```python
from build123d import *

# Parameters (mm, degrees)
F0_W     = 170
F0_H     = 170
F1_DEPTH = 40
F2_W     = 155
F2_H     = 113
F3_DEPTH = 17
F4_DEPTH = 24
F6_D     = 3.7973
F7_W     = 16.0088125554
F7_H     = 25.888455566
F7_W_2   = 40.4067277214
F7_H_2   = 12.8438859247
F7_W_3   = 24.2321552965
F7_H_3   = 26.0891397484
F7_W_4   = 19.8441686174
F7_H_4   = 32.3103985284
F8_DEPTH = 2


with BuildPart() as f1:
    # F0 (on Top) → F1 (new body)
    with BuildSketch(Plane.XY):
        Rectangle(F0_W, F0_H)
    extrude(amount=F1_DEPTH)

    # F2 (on face) → F3 (join)
    with BuildSketch(Plane.XY.offset(40)):
        with Locations((7.5, 1.5)):
            Rectangle(F2_W, F2_H)
    extrude(amount=F3_DEPTH)

    # F2 (on face) → F4 (cut)
    with BuildSketch(Plane.XY.offset(40)):
        Polygon((-70, 58), (-70, 85), (-85, 85), (-85, -85), (-70, -85), (-70, -55), align=None)
    extrude(amount=-F4_DEPTH, mode=Mode.SUBTRACT)

    # F6 (through all)
    with Locations(Plane(origin=(0, 0, 0), x_dir=(1, 0, 0), z_dir=(0, 0, -1))):
        with Locations((-78.65, -74.84), (78.83, -51.98), (78.83, 81.04), (-78.65, 81.04)):
            Hole(F6_D / 2)

    # F7 (on face) → F8 (join)
    with BuildSketch(Plane(origin=(0, 85, 0), x_dir=(-1, 0, 0), z_dir=(0, 1, 0))):
        with Locations((-71.7186613039, 17.3905782867)):
            Rectangle(F7_W, F7_H)
        with Locations((-35.5920631724, 10.868293466)):
            Rectangle(F7_W_2, F7_H_2)
        with Locations((7.3542475339, 17.4909203779)):
            Rectangle(F7_W_3, F7_H_3)
        with Locations((55.5439972199, 20.6015497679)):
            Rectangle(F7_W_4, F7_H_4)
    extrude(amount=F8_DEPTH)


solid = f1.part
```
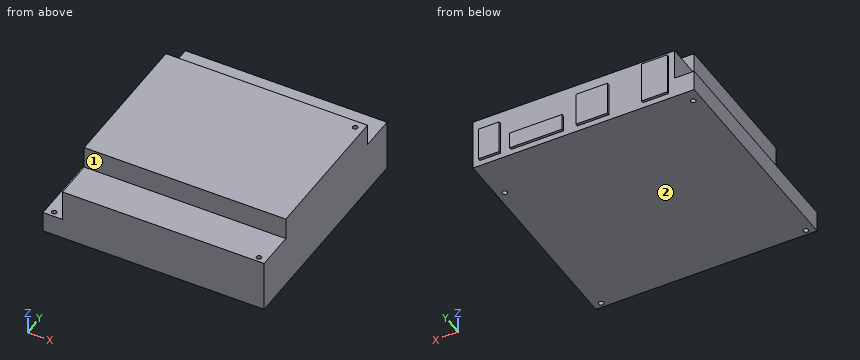
Can you work these out from the model? Positions are in its coordinate system, mm. Face numbers are marked on the shaded views. A direction names the side the tool comes from. Coordinates: 2 decimals unless noted, no trailing zeros. Loops run counter-clockwise (first coordinate to the right, second up) from the corner with the lowest first, then second, coordinate; pieces in that order, holes last. Notation, with made-up numbers: (-14.5, 58.25) -> (-3.5, 58.25) arc R29 cw to (-3.5, 88.25) -> close; hole circle Ø4 at (64.5, -8). An arc over 180 degrees is marked (long way). Put each result on its own line as item: value. Start each with the question number.
Q1. I want a section at A-A (z = 22). Write out the boundary of the cut face in (x, y).
Q2. For the marked faces 1 and 2, which set-ups out of +Z, -Z, +X, -X, +Y, -Y let a thin tool reach every point of the face, with its end or its side?
Q3. I want a section at B-B (y = -4). Write out the boundary of the cut face in (x, z).
Q4. If I drill on line 1 (Y direction, x = -78.65, z = 9.75); line 2 (X direction, y = -81, z = 11); line 3 (Y direction, x = 78.83, z = 28), over which ranges is the centre line in solid material (lowest first)? Write a range as [from, to].
Q5. I'm going to push flat-ended pins straight in: P1, Ø1.6, axis at y = 85.5, z = 13.5, coming from the -X side; P2, Ø1.6, axis at x = 71.5, y = 86.5, coming from the +Z side; P3, Ø8.5, axis at x = -8, z = 52, coming from the +Y side; P4, Ø1, axis at y = 86, z = 13.5, coming from the +X side. Where does each tip first touch, or does it pass through?
Q6. I want a section at C-C (y = -70.5). Write out the boundary of the cut face in (x, z).
Taken from the geometry:
1. outline: (-70, -85) -> (85, -85) -> (85, 85) -> (79.72, 85) -> (79.72, 87) -> (63.71, 87) -> (63.71, 85) -> (4.76, 85) -> (4.76, 87) -> (-19.47, 87) -> (-19.47, 85) -> (-45.62, 85) -> (-45.62, 87) -> (-65.47, 87) -> (-65.47, 85) -> (-70, 85) -> close; hole circle Ø3.8 at (78.83, -81.04); hole circle Ø3.8 at (78.83, 51.98)
2. face 1: +Z, +X, -X, -Y
2. face 2: -Z, +X, -X, +Y, -Y
3. outline: (-85, 0) -> (85, 0) -> (85, 57) -> (-70, 57) -> (-70, 16) -> (-85, 16) -> close
4. line 1: y = [-85, -82.94], [-79.14, 72.94], [76.74, 85]
4. line 2: x = [-85, -80.55], [-76.75, 76.93], [80.73, 85]
4. line 3: y = [-85, -82.94], [-79.14, 50.08], [53.88, 87]
5. P1: stops at x = -85
5. P2: stops at z = 30.33
5. P3: stops at y = 58
5. P4: stops at x = 79.72
6. outline: (-85, 0) -> (85, 0) -> (85, 40) -> (-70, 40) -> (-70, 16) -> (-85, 16) -> close
